Here's the drawing with two shaded views (mm, measured from the low corner). I have some questions. Coordinates: 2 decimals unless noted, no trailing zeros. Write each loop counter-clockwise with the first axis right and the second up, starting at its lowest first coordinate (ties: lowest second). Pieces come first, ordered by that corner, then holes.
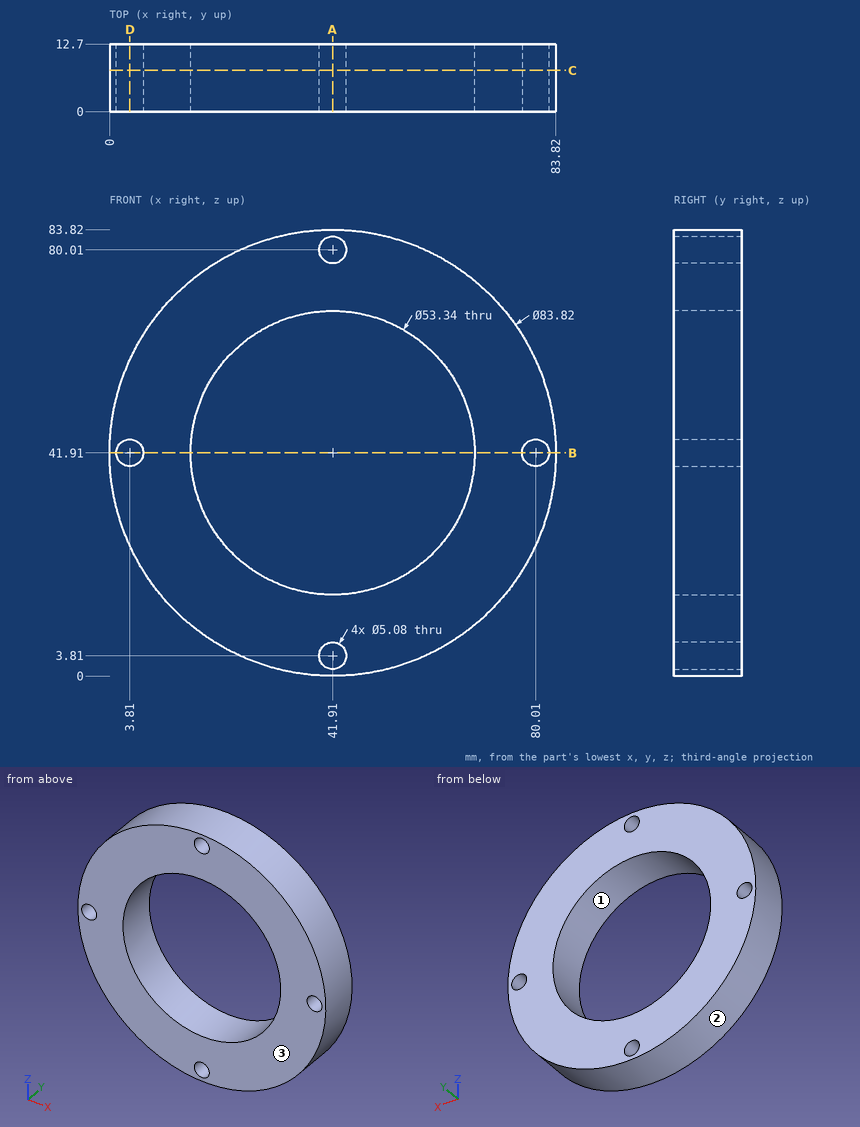
Item 1: If I drill on line 1 along X through (y, z) = (11, 42); line 2 along X through (y, z) = (4, 40); line 3 along X through (y, z) = (4.75, 66.5), over which ranges is the centre line in solid material (lowest first)?
Item 2: I want a section at C-C, the plane y = 7.75. List the corners of the cut face in (x, z) for me, then the cut area to 3 significant figures.
Item 3: I want a section at A-A, the plane x = 41.91. List the corners of the cut face in (y, z) for me.
Item 4: I want a section at D-D, the plane x = 3.81. List the corners of the cut face in (y, z) for me.
Item 5: I want a section at B-B, the plane z = 41.91. List the corners of the cut face in (x, y) for me.
Item 6: Will these pins go through, and if not, where does the flat tip stop? pin 1 Ø5 at (x, y) = (22.5, 9) entering from +Z; pin 2 Ø4 at (x, y) = (68, 8.5) entering from -Z; pin 3 Ø1.5 at (y, z) = (10.5, 56) entering from -X.
Item 7: If we mould it in two halves opening along X, with no side actions, what happens to the marked faces 1, 2 and 3? For each: released by +X, released by -X, zero draft, split by the parting line, or undercut.
Taken from the geometry:
1. line 1: x = 0 to 1.27, 6.35 to 15.24, 68.58 to 77.47, 82.55 to 83.82
1. line 2: x = 0.04 to 2.14, 5.48 to 15.31, 68.51 to 78.34, 81.68 to 83.78
1. line 3: x = 7.97 to 31.58, 52.24 to 75.85
2. outline: circle Ø83.82 at (41.91, 41.91); hole circle Ø5.08 at (3.81, 41.91); hole circle Ø53.34 at (41.91, 41.91); hole circle Ø5.08 at (41.91, 3.81); hole circle Ø5.08 at (41.91, 80.01); hole circle Ø5.08 at (80.01, 41.91)
2. area: 3,200 mm2
3. outline: (0, 0) - (12.7, 0) - (12.7, 1.27) - (0, 1.27) - close; (0, 6.35) - (12.7, 6.35) - (12.7, 15.24) - (0, 15.24) - close; (0, 68.58) - (12.7, 68.58) - (12.7, 77.47) - (0, 77.47) - close; (0, 82.55) - (12.7, 82.55) - (12.7, 83.82) - (0, 83.82) - close
4. outline: (0, 24.45) - (12.7, 24.45) - (12.7, 39.37) - (0, 39.37) - close; (0, 44.45) - (12.7, 44.45) - (12.7, 59.37) - (0, 59.37) - close
5. outline: (0, 0) - (1.27, 0) - (1.27, 12.7) - (0, 12.7) - close; (6.35, 0) - (15.24, 0) - (15.24, 12.7) - (6.35, 12.7) - close; (68.58, 0) - (77.47, 0) - (77.47, 12.7) - (68.58, 12.7) - close; (82.55, 0) - (83.82, 0) - (83.82, 12.7) - (82.55, 12.7) - close
6. pin 1: stops at z = 80.26
6. pin 2: stops at z = 7.62
6. pin 3: stops at x = 2.18
7. face 1: undercut
7. face 2: split by the parting line
7. face 3: zero draft
